Verification items for the finished model (mm, model axes). A direction names the side the tool comes from. Give positions to 0.01 mm unless a question says otherwise; leave off trailing zeros. Write each loop counter-clockwise with the first axis right and the second up, starting at its lowest first coordinate (ties: lowest second). Pieces come first, ordered by that corner, then holes. Notation, with made-up numbers: (15, 15.5) -> (57, 15.5) arc R6 cw to (57, 19.5) -> close; hole circle Ø5 at (73, -20). An arc over 180 degrees is marked (long way). Write item = value, one per line.
from build123d import *

# Parameters (mm, degrees)
F1_DEPTH = 0.8
F2_R     = 0.9
F2_R_2   = 1
F2_W     = 6.9
F2_H     = 0.2
F3_DEPTH = 1.9
F4_R     = 0.1


with BuildPart() as f1:
    # F0 (on Top) → F1 (new body)
    with BuildSketch(Plane.XY):
        with BuildLine():
            Line((0, 0.325), (0, 0))
            Line((0, 0), (7.1, 0))
            Line((7.1, 0), (7.1, 0.325))
            ThreePointArc((7.1, 0.325), (6.8, 0.625), (7.1, 0.925))
            Line((7.1, 0.925), (7.1, 1.425))
            ThreePointArc((7.1, 1.425), (6.8, 1.725), (7.1, 2.025))
            Line((7.1, 2.025), (7.1, 2.35))
            Line((7.1, 2.35), (0, 2.35))
            Line((0, 2.35), (0, 2.025))
            ThreePointArc((0, 2.025), (0.2121320344, 1.9371320344), (0.3, 1.725))
            ThreePointArc((0.3, 1.725), (0.2121320344, 1.5128679656), (0, 1.425))
            Line((0, 1.425), (0, 0.925))
            ThreePointArc((0, 0.925), (0.2121320344, 0.8371320344), (0.3, 0.625))
            ThreePointArc((0.3, 0.625), (0.2121320344, 0.4128679656), (0, 0.325))
        make_face()
    extrude(amount=F1_DEPTH)

    # F2 (on face) → F3 (join)
    with BuildSketch(Plane.XY.offset(0.8)):
        with BuildLine():
            Line((7, 2.35), (0.1, 2.35))
            Line((0.1, 2.35), (0.1, 2.0078427125))
            ThreePointArc((0.1, 2.0078427125), (0.3, 1.725), (0.1, 1.4421572875))
            Line((0.1, 1.4421572875), (0.1, 0.9078427125))
            ThreePointArc((0.1, 0.9078427125), (0.3, 0.625), (0.1, 0.3421572875))
            Line((0.1, 0.3421572875), (0.1, 0))
            Line((0.1, 0), (7, 0))
            Line((7, 0), (7, 0.3421572875))
            ThreePointArc((7, 0.3421572875), (6.8, 0.625), (7, 0.9078427125))
            Line((7, 0.9078427125), (7, 1.4421572875))
            ThreePointArc((7, 1.4421572875), (6.8, 1.725), (7, 2.0078427125))
            Line((7, 2.0078427125), (7, 2.35))
        make_face()
        with Locations((1.6234196955, 1.175)):
            Circle(F2_R, mode=Mode.SUBTRACT)
        with Locations((5.5034196955, 1.175)):
            Circle(F2_R_2, mode=Mode.SUBTRACT)
        with Locations((3.55, 2.45)):
            Rectangle(F2_W, F2_H)
        with Locations((3.55, -0.1)):
            Rectangle(F2_W, F2_H)
        with BuildLine():
            ThreePointArc((0.1, 0.3421572875), (0.3, 0.625), (0.1, 0.9078427125))
            Line((0.1, 0.9078427125), (0.1, 0.3421572875))
        make_face()
        with BuildLine():
            ThreePointArc((0.1, 1.4421572875), (0.3, 1.725), (0.1, 2.0078427125))
            Line((0.1, 2.0078427125), (0.1, 1.4421572875))
        make_face()
        with BuildLine():
            Line((7, 1.4421572875), (7, 2.0078427125))
            ThreePointArc((7, 2.0078427125), (6.8, 1.725), (7, 1.4421572875))
        make_face()
        with BuildLine():
            Line((7, 0.3421572875), (7, 0.9078427125))
            ThreePointArc((7, 0.9078427125), (6.8, 0.625), (7, 0.3421572875))
        make_face()
    extrude(amount=F3_DEPTH)

    # F4
    f4_edges = [f1.edges().sort_by_distance(p)[0] for p in [
        (0.1, 1.175, 2.7),
        (0.1, -0.2, 1.75),
        (0.1, 2.55, 1.75),
        (7, -0.2, 1.75),
        (7, 2.55, 1.75),
        (3.55, 2.55, 2.7),
        (3.55, -0.2, 2.7),
        (7, 1.175, 2.7),
    ]]
    fillet(f4_edges, radius=F4_R)


solid = f1.part
Item 1: Material ranges on line 1 (X direction, y = 1.85, z = 2.15); line 2 (X direction, y = 1.6, z = 1.15); line 3 (Y direction, x = 2.25, z = 0.75), recorded low to high.
Response values:
line_1 = 0.1 to 1.03, 2.22 to 4.77, 6.24 to 7
line_2 = 0.1 to 0.83, 2.42 to 4.6, 6.41 to 7
line_3 = 0 to 2.35
Item 2: Set-up check for faces 1 (the flat face through (0.1, 1, 2)), 2 (the flat face through (7, 1, 2)), 3 (the cylindrical face through (6.457, 1.475, 1.737)): record each of +Z, -Z, +X, -X, +Y, -Y from which the full face is reachable in a straight line by a thin tool's end or side.
Response values:
face_1 = +Z, -X, +Y, -Y
face_2 = +Z, +X, +Y, -Y
face_3 = +Z
Item 3: Sectioned sample at D-D on z = 0.9. Record the cut outline in (x, y) (3 decimals).
Response values:
outline = (0.1, -0.1) arc R0.1 ccw to (0.2, -0.2) -> (6.9, -0.2) arc R0.1 ccw to (7, -0.1) -> (7, 2.45) arc R0.1 ccw to (6.9, 2.55) -> (0.2, 2.55) arc R0.1 ccw to (0.1, 2.45) -> close; hole circle Ø1.8 at (1.623, 1.175); hole circle Ø2 at (5.503, 1.175)
Item 4: Go/stop test with flat-tipped pins: P1, Ø0.9, axis at y = 1, z = 2, coming from the +X side; P2, Ø0.5, axis at y = 0.5, z = 1.5, coming from the -X side. Record where each tip stops, or that it passes through.
Response values:
P1 = 7
P2 = 0.1
Item 5: Sectioned sample at C-C on y = 1.85. Record the cut outline in (x, z).
Response values:
outline = (0.1, 0.8) -> (0.27, 0.8) -> (0.27, 0) -> (6.83, 0) -> (6.83, 0.8) -> (7, 0.8) -> (7, 2.6) arc R0.1 ccw to (6.9, 2.7) -> (6.24, 2.7) -> (6.24, 0.8) -> (4.77, 0.8) -> (4.77, 2.7) -> (2.22, 2.7) -> (2.22, 0.8) -> (1.03, 0.8) -> (1.03, 2.7) -> (0.2, 2.7) arc R0.1 ccw to (0.1, 2.6) -> close
Item 6: Sectioned sample at A-A on z = 0.6. Record the cut outline in (x, y) (3 decimals).
Response values:
outline = (0, 0) -> (7.1, 0) -> (7.1, 0.325) arc R0.3 cw to (7.1, 0.925) -> (7.1, 1.425) arc R0.3 cw to (7.1, 2.025) -> (7.1, 2.35) -> (0, 2.35) -> (0, 2.025) arc R0.3 cw to (0, 1.425) -> (0, 0.925) arc R0.3 cw to (0, 0.325) -> close
Item 7: Mould release check, pull along Y, two halves, no side actions. Record for faces 4 (the flat face through (4, 2.55, 2)), 5 (the cylindrical face through (0.909, 0.627, 1.737)), 6 (the flat face through (4, 1, 2.7)), 7 (the flat face through (4, -0.2, 2)): +Y half, -Y half, draft (parallel to the pull), parting line (faces both ways), or undercut.
Response values:
face_4 = +Y half
face_5 = undercut
face_6 = draft
face_7 = -Y half
Item 8: Sectioned sample at B-B on x = 4. Record the cut outline in (y, z), then the cut area to 3 significant figures.
Response values:
outline = (-0.2, 0.8) -> (0, 0.8) -> (0, 0) -> (2.35, 0) -> (2.35, 0.8) -> (2.55, 0.8) -> (2.55, 2.6) arc R0.1 ccw to (2.45, 2.7) -> (-0.1, 2.7) arc R0.1 ccw to (-0.2, 2.6) -> close
area = 7.10 mm^2
